Autodesk Inventor part; units mm, degrees
ref_plane "Work Plane1" through (609.6, 0, 0) normal (1, 0, 0) x (0, 0, -1)
ref_plane "YZ Plane" through (0, 0, 0) normal (1, 0, 0) x (0, 1, 0)
ref_plane "XZ Plane" through (0, 0, 0) normal (0, 1, 0) x (-1, 0, 0)
sketch "Sketch1" plane through (0, 0, 0) normal (1, 0, 0) x (0, 1, 0)
  line L0 (0, 0) -> (25.4, 0) construction
  line L1 (25.4, 0) -> (25.4, -1.5875) construction
  line L2 (25.4, -1.5875) -> (0, -1.5875) construction
  line L3 (0, -1.5875) -> (0, 0) construction
  circle A0 centre (4.7625, 3.175) radius 4.7625 construction
  line L4 (25.4, 0) -> (25.4, -1.5875)
  line L5 (25.4, -1.5875) -> (4.7625, -1.5875)
  line L6 (25.4, 0) -> (8.3123, 0)
  arc A1 (8.3123, 0) -> (4.7625, -1.5875) centre (4.7625, 3.175) ccw
  dimension "d0" = 25.4
  dimension "d1" = 1.5875
  dimension "d2" = 9.525
  dimension "d3" = 4.7625
  dimension "d4" = 3.175
extrude "Extrusion1" add sketch "Sketch1" along normal blind 635
sketch "Sketch2" plane through (635, 0, 0) normal (1, 0, 0) x (0, 0, -1)
  arc A0 (0, 8.3123) -> (1.5875, 4.7625) centre (-3.175, 4.7625) ccw
  circle A1 centre (-3.175, 4.7625) radius 3.175
  point P0 (0, 0)
  dimension "d7" = 6.35
extrude "Extrusion2" cut sketch "Sketch2" against normal blind 635
sketch "Sketch4" plane through (635, 25.4, -1.5875) normal (0, 0, -1) x (-1, 0, 0)
  line L0 (635, 0) -> (0, 0)
  line L1 (0, -20.6375) -> (0, 0)
  point P0 (0, -17.0877)
  point P1 (635, -25.4)
  point P2 (12.7, -9.525)
  dimension "d15" = 9.525
  dimension "d16" = 12.7
hole "Hole1" at (622.3, 15.875, -1.5875) direction (0, 0, 1) diameter 6.35 end through all
pattern_linear "Rectangular Pattern2" count 25 spacing 25.4 along (-1, 0, 0) of "Hole1"
ref_plane "Work Plane1" through (609.6, 0, 0) normal (1, 0, 0) x (0, 0, -1)
sketch "Sketch5" plane through (609.6, 0, 0) normal (1, 0, 0) x (0, 0, -1)
  circle A0 centre (-3.175, 4.7625) radius 3.175
  line L0 (1.5875, 25.4) -> (0, 25.4)
  line L1 (0, 25.4) -> (0, 8.3123)
  arc A1 (0, 8.3123) -> (1.5875, 4.7625) centre (-3.175, 4.7625) ccw
  line L2 (1.5875, 4.7625) -> (1.5875, 25.4)
  line L3 (0, 8.3123) -> (1.5875, 8.3123)
  line L4 (1.5875, 4.7625) -> (1.5875, 25.4)
  line L5 (1.5875, 8.3123) -> (1.5875, 4.7625)
  arc A2 (0, 8.3123) -> (1.5875, 4.7625) centre (-3.175, 4.7625) ccw
  point P0 (0, 0)
extrude "Extrusion4" cut sketch "Sketch5" against normal blind 25.4 contours L2 A1 L3
pattern_linear "Rectangular Pattern3" count 12 spacing 50.8 along (-1, 0, 0) of "Extrusion4"
properties part number "continuous hinge bottom"
Model file for the job. Use its own axes, mm. Coordinates: 2 decimals unless noted, no trailing zeros. Return JSON: item names as keys, results as strings.
Item 1: Wall check: line 1 along Y through (x, z) = (270, 3); line 2 along Y through (x, z) = (495.3, -1.2); line 3 along Z through (x, y) = (453, 8.5). Give the ranges that are in metal, low to high. Write a range as from..to.
Model answer:
{"line 1": "y = 0..1.59, 7.93..9.52", "line 2": "y = 8.31..12.7, 19.05..25.4", "line 3": "z = -1.59..0"}
Item 2: Slice it at A-A (z = 2.5). Count the separate pieces of the cut face and the enclosed holes in it, then the cut area to 3 significant figures.
Model answer:
{"separate pieces": "26", "enclosed holes": "0", "area": "1,060 mm²"}
Item 3: Pin check, flat tips, straight feed: P1, Ø5.5, axis at x = 38.1, y = 15.875, coming from the +Z side; P2, Ø5, axis at y = 3, z = 4.5, coming from the -X side; P3, Ø3, axis at x = 313, z = 6, coming from the +Y side; P4, Ø1.3, axis at x = 541.5, z = -0.5, coming from the -Y side. Stop position of each tip, or through.
Model answer:
{"P1": "passes through", "P2": "stops at x = 0", "P3": "stops at y = 9.34", "P4": "stops at y = 8.31"}
